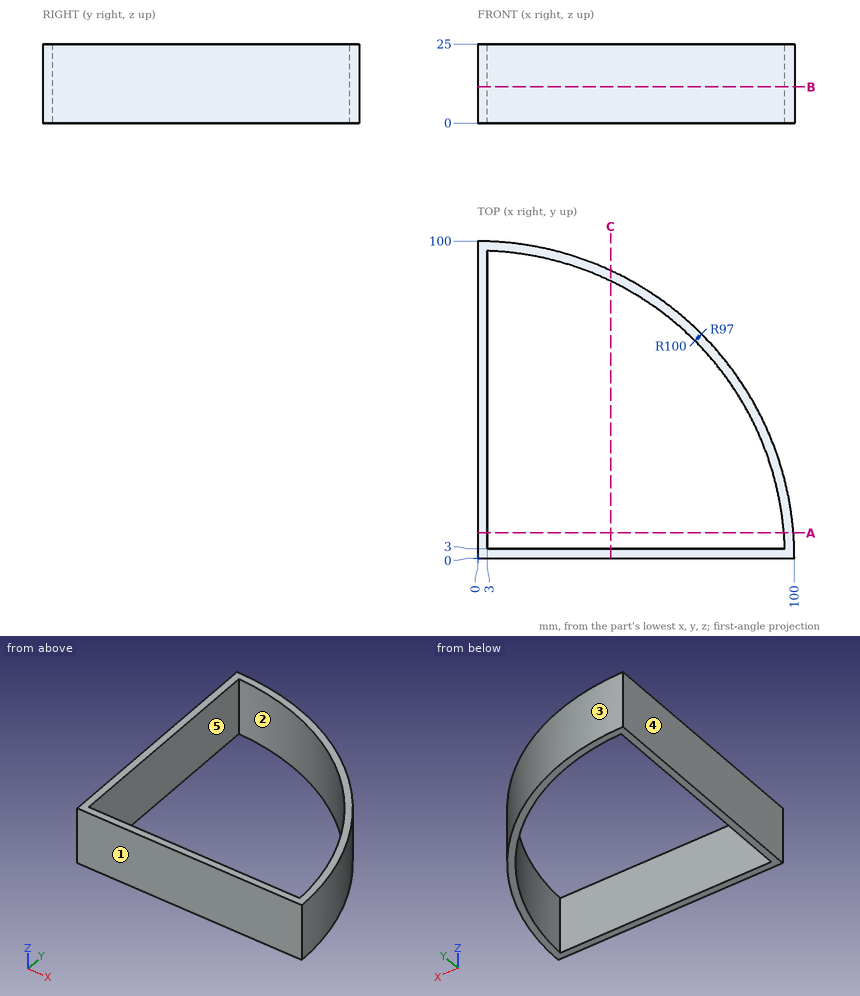
Here's the drawing with two shaded views (mm, measured from the low corner). I have some questions. A direction names the side the tool comes from. Give positions to 0.01 mm unless a question says otherwise; leave off trailing zeros. Loops run counter-clockwise (first coordinate to the right, second up) from the corner with the lowest first, then second, coordinate; pieces in that order, holes last. Notation, with made-up numbers: M 11.5,18.5 L 67.5,18.5 A26 cw 67.5,36.5 Z; hole C 70,73 d5. An arc over 180 degrees is marked long. Answer in a Markdown table with one row per item.
1. Suppose I cut it at C-C on x = 42. Write out the boundary of the cut face in (y, z).
Taken from the geometry:
| item | result |
|---|---|
| outline | M 0,0 L 3,0 L 3,25 L 0,25 Z; M 87.44,0 L 90.75,0 L 90.75,25 L 87.44,25 Z |
2. Which directions (+Z, -Z, +X, -X, +Y, -Y) give clear straight access to the entire face, cutting with the end or side of a thin tool? Please do the marked faces 4 and 5.
Taken from the geometry:
| item | result |
|---|---|
| face 4 | +Z, -Z, -X, +Y, -Y |
| face 5 | +Z, -Z |
3. If I drill on line 1 along X through (y, z) = (45.5, 19); line 2 along Y through (x, z) = (51.5, 17); line 3 along Y through (x, z) = (57.5, 6.75), over which ranges is the centre line in solid material (lowest first)?
Taken from the geometry:
| item | result |
|---|---|
| line 1 | x = 0 to 3, 85.67 to 89.05 |
| line 2 | y = 0 to 3, 82.2 to 85.72 |
| line 3 | y = 0 to 3, 78.12 to 81.82 |
4. Thinking about a two-plate mould opening in X: for the marked faces 1, 2 and 3, which applies, released by +X, released by -X, zero draft, split by the parting line, or undercut?
Taken from the geometry:
| item | result |
|---|---|
| face 1 | zero draft |
| face 2 | undercut |
| face 3 | released by +X |
5. Suppose I cut it at A-A on y = 8. Write out the boundary of the cut face in (x, z), plus the area to 3 significant figures.
Taken from the geometry:
| item | result |
|---|---|
| outline | M 0,0 L 3,0 L 3,25 L 0,25 Z; M 96.67,0 L 99.68,0 L 99.68,25 L 96.67,25 Z |
| area | 150 mm² |
6. For pin 1 Ø8 at (x, z) = (50, 22.5) entering from +Y; pin 2 Ø7.5 at (x, z) = (64, 7) entering from +Y; pin 3 Ø6 at (y, z) = (31, 12.5) entering from +X, each with a flat end and sliding along its axis, tell me the tip position at first contact or that it passes through.
Taken from the geometry:
| item | result |
|---|---|
| pin 1 | stops at y = 88.79 |
| pin 2 | stops at y = 79.81 |
| pin 3 | stops at x = 96 |
7. Suppose I cut it at B-B on z = 11.5. Write out the boundary of the cut face in (x, y), plus the area to 3 significant figures.
Taken from the geometry:
| item | result |
|---|---|
| outline | M 0,0 L 100,0 A100 ccw 0,100 Z; hole M 3,3 L 96.95,3 A97 ccw 3,96.95 Z |
| area | 1,040 mm² |
